Autodesk Inventor part; units mm, degrees
ref_plane "YZ Plane" through (0, 0, 0) normal (1, 0, 0) x (0, 1, 0)
ref_plane "XZ Plane" through (0, 0, 0) normal (0, 1, 0) x (-1, 0, 0)
ref_plane "XY Plane" through (0, 0, 0) normal (0, 0, 1) x (1, 0, 0)
sketch "Sketch1" plane through (0, 0, 0) normal (0, 1, 0) x (-1, 0, 0)
  line L0 (0, 0) -> (-12, 0)
  line L1 (-12, 0) -> (-12, -12)
  line L2 (-12, -12) -> (0, -12)
  line L3 (0, -12) -> (0, 0)
  dimension "d0" = 12
  dimension "d1" = 12
extrude "Extrusion1" add sketch "Sketch1" along normal blind 7
sketch "Sketch2" plane through (0, 0, -12) normal (-1, 0, 0) x (0, 0, 1)
  line L0 (12, 0) -> (0, 0)
  line L1 (0, 0) -> (12, 0)
  line L2 (12, 0) -> (12, 19)
  line L3 (12, 19) -> (0, 19)
  line L4 (0, 19) -> (0, 0)
  dimension "d4" = 12
  dimension "d5" = 19
extrude "Extrusion2" add sketch "Sketch2" along normal blind 7
sketch "Sketch3" plane through (0, 0, -12) normal (1, 0, 0) x (0, 0, -1)
  circle A0 centre (-6, 14.5) radius 3.25 construction
  line L0 (-12, 19) -> (0, 19) construction
  line L1 (-12, 7) -> (-12, 19) construction
  line L2 (-2.75, 14.5) -> (-4.375, 11.6854)
  line L3 (-4.375, 11.6854) -> (-7.625, 11.6854)
  line L4 (-7.625, 11.6854) -> (-9.25, 14.5)
  line L5 (-9.25, 14.5) -> (-7.625, 17.3146)
  line L6 (-7.625, 17.3146) -> (-4.375, 17.3146)
  line L7 (-4.375, 17.3146) -> (-2.75, 14.5)
  point P0 (-12, 0)
  dimension "d8" = 6.5
  dimension "d9" = 4.5
  dimension "d10" = 6
extrude "Extrusion3" cut sketch "Sketch3" against normal blind 4
sketch "Sketch4" plane through (0, 7, 0) normal (0, 1, 0) x (1, 0, 0)
  circle A0 centre (7.5, 6) radius 3.25 construction
  line L0 (12, 0) -> (12, 12) construction
  line L1 (12, 12) -> (0, 12) construction
  line L2 (0, 0) -> (12, 0) construction
  line L3 (7.5, 9.25) -> (10.3146, 7.625)
  line L4 (10.3146, 7.625) -> (10.3146, 4.375)
  line L5 (10.3146, 4.375) -> (7.5, 2.75)
  line L6 (7.5, 2.75) -> (4.6854, 4.375)
  line L7 (4.6854, 4.375) -> (4.6854, 7.625)
  line L8 (4.6854, 7.625) -> (7.5, 9.25)
  dimension "d13" = 6.5
  dimension "d14" = 4.5
  dimension "d15" = 6
  dimension "d16" = 12
extrude "Extrusion4" cut sketch "Sketch4" against normal blind 4
fillet "Fillet1" radius 4 1 edges at (0, 7, -6)
sketch "Sketch7" plane through (0, 0, -12) normal (1, 0, 0) x (0, 0, -1)
  line L0 (-9.25, 14.5) -> (-7.625, 17.3146) construction
  line L1 (-4.375, 17.3146) -> (-2.75, 14.5) construction
  line L2 (-9.25, 14.5) -> (-2.75, 14.5) construction
  line L3 (-7.625, 17.3146) -> (-4.375, 17.3146) construction
  line L4 (-4.375, 11.6854) -> (-7.625, 11.6854) construction
  line L5 (-4.375, 17.3146) -> (-7.625, 11.6854) construction
  circle A0 centre (-6, 14.5) radius 1.7
  point P0 (-12, 0)
  dimension "d24" = 3.4
extrude "Extrusion7" cut sketch "Sketch7" against normal through all
sketch "Sketch8" plane through (0, 7, 0) normal (0, 1, 0) x (1, 0, 0)
  line L0 (7.5, 9.25) -> (10.3146, 7.625) construction
  line L1 (4.6854, 4.375) -> (4.6854, 7.625) construction
  line L2 (10.3146, 7.625) -> (4.6854, 4.375) construction
  line L3 (4.6854, 7.625) -> (7.5, 9.25) construction
  line L4 (10.3146, 7.625) -> (10.3146, 4.375) construction
  line L5 (4.6854, 7.625) -> (10.3146, 4.375) construction
  circle A0 centre (7.5, 6) radius 1.7
  point P0 (0, 0)
  dimension "d27" = 3.4
extrude "Extrusion8" cut sketch "Sketch8" against normal through all
properties part number "wheel box lid bracket"
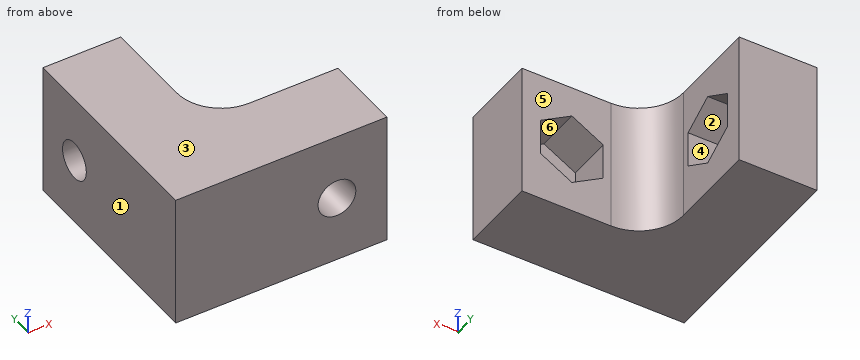
Part model, mm, in its own coordinate system. Face numbers are marked on the shaded views. A direction names the side the tool comes from. Round coordinates to 2 decimals unless told otherwise and drop trailing zeros. Write each loop counter-clockwise with the first axis right and the second up, starting at its lowest first coordinate (ties: lowest second). Pieces come first, ordered by that corner, then holes. Notation, with made-up numbers: (67.25, 28) - (119.25, 28) arc R15 ccw to (119.25, 44) - close; hole circle Ø11 at (-21, -10.75). An arc over 180 degrees is marked (long way). Use CSV: the item, a comma, the result in double quotes.
Item 1: Pull direction Z, two halves, no side cores. Call the marked faces 1, 2 and 3: pulls with the +Z half, pulls with the -Z half, needs draft (parallel to the pull), parting line crosses it, or undercut.
Results list:
face 1,"needs draft"
face 2,"undercut"
face 3,"pulls with the +Z half"
Item 2: Tool access for the marked faces 4, 5 and 6: list every direction of +Z, -Z, +X, -X, +Y, -Y with a clear straight run to the whole face (end or side of a thin tool).
Results list:
face 4,"+X"
face 5,"+Z, -Z, +X, +Y"
face 6,"+Y"
Item 3: Flat gauge pins, fed straight in: P1, Ø3, axis at x = 8, z = -5.5, coming from the +Y side; P2, Ø3, axis at x = 5.5, z = -8.5, coming from the +Y side; P3, Ø2, axis at y = 14.5, z = -6, coming from the -X side; P4, Ø4, axis at y = 16, z = -7, coming from the +X side. Where does each tip first touch, or does it go through?
Results list:
P1,"stops at y = 3"
P2,"stops at y = 7"
P3,"passes through"
P4,"stops at x = 0"
Item 4: Slice it at D-D, the plane y = 8.5. Write the cut outline in (x, z), then the cut area to 3 significant figures.
Results list:
outline,"(-7, -12) - (0.88, -12) - (0.88, 0) - (-7, 0) - close"
area,"94.5 mm²"
Item 5: Slice it at A-A, the plane z = -6. Write the cut outline in (x, y), then the cut area to 3 significant figures.
Results list:
outline,"(-7, 0) - (5.8, 0) - (5.8, 3) - (4.69, 3) - (4.69, 7) - (4, 7) arc R4 cw to (0, 11) - (0, 11.69) - (-4, 11.69) - (-4, 12.8) - (-7, 12.8) - close; (-7, 16.2) - (-4, 16.2) - (-4, 17.31) - (0, 17.31) - (0, 19) - (-7, 19) - close; (9.2, 0) - (12, 0) - (12, 7) - (10.31, 7) - (10.31, 3) - (9.2, 3) - close"
area,"155 mm²"
Item 6: Wall check: L1, parallel to X at y = 2.25, z = -6; L2, parallel to Z at x = 7.5, y = 0.85; L3, parallel to Y at x = -5.15, z = -6. Give the ranges that are in metal, low to high.
Results list:
L1,"x = -7 to 5.8, 9.2 to 12"
L2,"z = -12 to -7.7, -4.3 to 0"
L3,"y = 0 to 12.8, 16.2 to 19"
Item 7: Slice it at C-C, the plane z = -1.75. Write the cut outline in (x, y).
Results list:
outline,"(-7, 0) - (12, 0) - (12, 7) - (4, 7) arc R4 cw to (0, 11) - (0, 19) - (-7, 19) - close"
Item 8: Slice it at B-B, the plane x = -1.5. Write the cut outline in (y, z) (3 decimals), then the cut area to 3 significant figures.
Results list:
outline,"(0, -12) - (19, -12) - (19, 0) - (0, 0) - close; hole (11.685, -7.625) - (14.5, -9.25) - (17.315, -7.625) - (17.315, -4.375) - (14.5, -2.75) - (11.685, -4.375) - close"
area,"201 mm²"
